```python
from build123d import *

# Parameters (mm, degrees)
ESQUISSE1_R             = 15.25
BOSS_EXTRU_1_DEPTH      = 90
ESQUISSE2_R             = 11
ENL_V_MAT_EXTRU_1_DEPTH = 7
ESQUISSE3_R             = 9
ENL_V_MAT_EXTRU_2_DEPTH = 5


with BuildPart() as part:
    # Esquisse1 → Boss.-Extru.1 (new body)
    with BuildSketch(Plane.XY):
        with Locations(Location((0, 0, 0), (0, 0, 180))):
            Circle(ESQUISSE1_R)
    extrude(amount=BOSS_EXTRU_1_DEPTH)

    # Esquisse2 → Enlèv. mat.-Extru.1 (cut)
    with BuildSketch(Plane.XY.offset(90)):
        Circle(ESQUISSE2_R)
    enl_v_mat_extru_1 = extrude(amount=-ENL_V_MAT_EXTRU_1_DEPTH, mode=Mode.SUBTRACT)

    # Esquisse3 → Enlèv. mat.-Extru.2 (cut)
    with BuildSketch(Plane.XY.offset(83)):
        Circle(ESQUISSE3_R)
    enl_v_mat_extru_2 = extrude(amount=-ENL_V_MAT_EXTRU_2_DEPTH, mode=Mode.SUBTRACT)

    # Symétrie1: Enlèv. mat.-Extru.1, Enlèv. mat.-Extru.2 across plane
    add(enl_v_mat_extru_1.mirror(Plane.XY.offset(45)), mode=Mode.SUBTRACT)
    add(enl_v_mat_extru_2.mirror(Plane.XY.offset(45)), mode=Mode.SUBTRACT)


solid = part.part
```
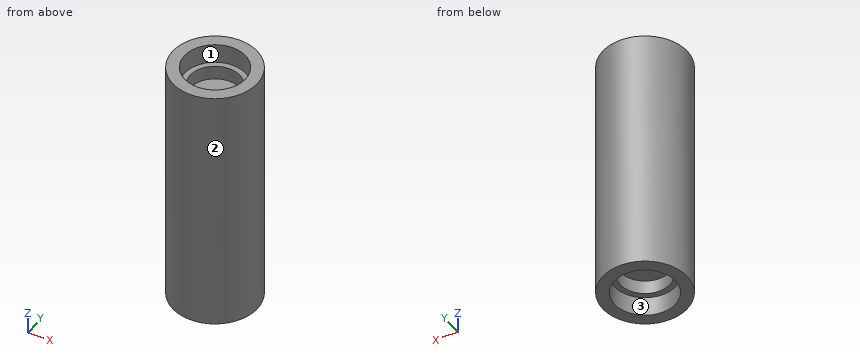
Check sheet for the modelled part. Datum: model origin and axes. Units: mm. Face numbers are marked on the shaded views. Coordinates: 2 decimals unless noted, no trailing zeros. Loops run counter-clockwise (first coordinate to the right, second up) from the corner with the lowest first, then second, coordinate; pieces in that order, holes last. Notation, with made-up numbers: M -29.75,-25 L -18.75,-25 A25 cw -18.75,5 Z; hole C 38,83 d10. An arc over 180 degrees is marked long. Answer as a JSON object with one key per item and string values.
1. Sectioned sample at A-A on y = 0. Record the cut outline in (x, z).
Outcome:
{"outline": "M -15.25,0 L -11,0 L -11,7 L -9,7 L -9,12 L 9,12 L 9,7 L 11,7 L 11,0 L 15.25,0 L 15.25,90 L 11,90 L 11,83 L 9,83 L 9,78 L -9,78 L -9,83 L -11,83 L -11,90 L -15.25,90 Z"}
2. Sectioned sample at C-C on z = 64. Record the cut outline in (x, y).
Outcome:
{"outline": "C 0,0 d30.5"}
3. Release check for a two-part mould opening along X. For the marked faces 1, 2 and 3 record: pulls with the +X half, pulls with the -X half, needs draft (parallel to the pull), parting line crosses it, or undercut.
Outcome:
{"face 1": "undercut", "face 2": "parting line crosses it", "face 3": "undercut"}
4. Depth check by flat-ended pin: P1, Ø1, axis at x = -2.5, y = -4.5, coming from the +Z side; P2, Ø4, axis at x = -6.5, y = 4.5, coming from the +Z side; P3, Ø3, axis at x = 8.5, z = 60, coming from the -Y side. Enter the tip coordinate at first touch or a pass-through.
Outcome:
{"P1": "z = 78", "P2": "z = 83", "P3": "y = -13.55"}
5. Scan lines: L1, parallel to Y at x = 0, z = 10; L2, parallel to Z at x = -1, y = -5.5; L3, parallel to Z at x = -8, y = 5. Record each from-to range of solid material in increasing order. Write a range as from..to.
Outcome:
{"L1": "-15.25..-9, 9..15.25", "L2": "12..78", "L3": "7..83"}
